Autodesk Inventor part; units mm, degrees
ref_plane "YZ Plane" through (0, 0, 0) normal (1, 0, 0) x (0, 1, 0)
ref_plane "XZ Plane" through (0, 0, 0) normal (0, 1, 0) x (-1, 0, 0)
ref_plane "XY Plane" through (0, 0, 0) normal (0, 0, 1) x (1, 0, 0)
sketch "Sketch1" plane through (0, 0, 0) normal (0, 0, 1) x (1, 0, 0)
  line L0 (0, 0) -> (-42.291, 0)
  line L1 (-42.291, 0) -> (-42.291, 42.291)
  line L2 (-42.291, 42.291) -> (0, 42.291)
  line L3 (0, 42.291) -> (0, 0)
  dimension "d0" = 42.291
  dimension "d1" = 42.291
extrude "Extrusion1" add sketch "Sketch1" along normal blind 42.291
sketch "Sketch2" plane through (0, 0, 42.291) normal (0, 0, 1) x (1, 0, 0)
  line L0 (0, 42.291) -> (-42.291, 42.291)
  line L1 (-42.291, 42.291) -> (-42.291, 0)
  line L2 (-42.291, 0) -> (0, 0)
  line L3 (0, 0) -> (0, 42.291)
  line L4 (-5.6515, 5.6515) -> (-36.6395, 5.6515)
  line L5 (-36.6395, 5.6515) -> (-36.6395, 36.6395)
  line L6 (-36.6395, 36.6395) -> (-5.6515, 36.6395)
  line L7 (-5.6515, 36.6395) -> (-5.6515, 5.6515)
  line L8 (-5.6515, 5.6515) -> (-36.6395, 36.6395) construction
  line L9 (-36.6395, 5.6515) -> (-5.6515, 36.6395) construction
  circle A0 centre (-5.6515, 5.6515) radius 2.794
  circle A1 centre (-36.6395, 5.6515) radius 2.794
  circle A2 centre (-36.6395, 36.6395) radius 2.794
  circle A3 centre (-5.6515, 36.6395) radius 2.794
  point P0 (-21.1455, 21.1455)
  dimension "d4" = 30.988
  dimension "d5" = 30.988
  dimension "d8" = 5.588
  dimension "d9" = 5.588
  dimension "d10" = 5.588
  dimension "d11" = 5.588
extrude "Extrusion2" cut sketch "Sketch2" against normal blind 68.834 contours A1 L5 L4 | L4 L5 A1 | A0 L7 L4 | L4 L7 A0 | A2 L6 L5 | L5 L6 A2 | A3 L6 L7 | L7 L6 A3
sketch "Sketch3" plane through (0, 0, 42.291) normal (0, 0, 1) x (1, 0, 0)
  circle A0 centre (-5.6515, 5.6515) radius 2.794
  circle A1 centre (-5.6515, 36.6395) radius 2.794
  circle A2 centre (-36.6395, 5.6515) radius 2.794
  circle A3 centre (-36.6395, 36.6395) radius 2.794
  line L0 (0, 42.291) -> (-42.291, 42.291)
  line L1 (-42.291, 42.291) -> (-42.291, 0)
  line L2 (-42.291, 0) -> (0, 0)
  line L3 (0, 0) -> (0, 42.291)
  circle A4 centre (-21.1455, 21.1455) radius 2.5019
  dimension "d14" = 5.0038
extrude "Extrusion3" add sketch "Sketch3" along normal blind 24.003 contours A4
properties part number "Nema 17"
For this review, take the finished solid that the model builds, in its own axes (mm). A direction names the side the tool comes from. Give positions to 0.01 mm unless a question says otherwise; leave off trailing zeros. Write each loop counter-clockwise with the first axis right and the second up, starting at its lowest first coordinate (ties: lowest second). Pieces come first, ordered by that corner, then holes. Notation, with made-up numbers: (12.5, 66) -> (63.5, 66) arc R12 cw to (63.5, 74) -> close; hole circle Ø4 at (32, 54.25). An arc over 180 degrees is marked (long way). Use CSV: the item, a comma, the result in double quotes.
Q1. For P1, Ø1, axis at x = -18, z = 59.5, coming from the -Y side; P2, Ø10, axis at x = -36.5, y = 10.5, coming from the +Z side, all flat-tipped, find the tip position at first contact; note any pin that passes through.
Conclusion:
P1,"through"
P2,"z = 42.29"
Q2. Take a section at A-A, the plane x = -38. Write out the cut boundary in (y, z).
Conclusion:
outline,"(0, 0) -> (3.21, 0) -> (3.21, 42.29) -> (0, 42.29) -> close; (8.09, 0) -> (34.2, 0) -> (34.2, 42.29) -> (8.09, 42.29) -> close; (39.08, 0) -> (42.29, 0) -> (42.29, 42.29) -> (39.08, 42.29) -> close"
Q3. Take a section at D-D, the plane x = -15. Write out the cut boundary in (y, z).
Conclusion:
outline,"(0, 0) -> (42.29, 0) -> (42.29, 42.29) -> (0, 42.29) -> close"
Q4. To check wall thickness, follow probe 1 along X at (y, z) = (4, 19); probe 2 along X at (y, z) = (8, 32.5); probe 3 along Y at (x, z) = (-35, 12.5). State the ranges of each line that lie inside material, in increasing order. Write a range as [from, to].
Conclusion:
probe 1,"[-42.29, -38.89], [-34.39, -7.91], [-3.4, 0]"
probe 2,"[-42.29, -38.15], [-35.13, -7.17], [-4.14, 0]"
probe 3,"[0, 3.39], [7.91, 34.38], [38.9, 42.29]"
Q5. Take a section at B-B, the plane y = 7. Write out the cut boundary in (x, z).
Conclusion:
outline,"(-42.29, 0) -> (-39.09, 0) -> (-39.09, 42.29) -> (-42.29, 42.29) -> close; (-34.19, 0) -> (-8.1, 0) -> (-8.1, 42.29) -> (-34.19, 42.29) -> close; (-3.2, 0) -> (0, 0) -> (0, 42.29) -> (-3.2, 42.29) -> close"
Q6. Tool access review of faces 5 (the face through (-23.645, 21.035, 54.124)), 6 (the face through (0, 21, 21)): name each direction out of +Z, -Z, +X, -X, +Y, -Y from which nothing blocks a thin tool from reaching the whole face with its end or side.
Conclusion:
face 5,"+Z"
face 6,"+Z, -Z, +X, +Y, -Y"
Q7. Mouldability with a two-part tool opening along Y and no side actions: class faces 1 (the face through (-6.02, 39.41, 21.44)), 2 (the face through (-21, 0, 21)), 3 (the face through (-38.857, 3.951, 21.442)), 4 (the face through (-26, 21, 42.291)) as pulls with the +Y half, pulls with the -Y half, needs draft (parallel to the pull), parting line crosses it, or undercut.
Conclusion:
face 1,"undercut"
face 2,"pulls with the -Y half"
face 3,"undercut"
face 4,"needs draft"
Q8. Take a section at C-C, the plane z = 34. Write out the cut boundary in (x, y), then the cut area to 3 significant figures.
Conclusion:
outline,"(-42.29, 0) -> (0, 0) -> (0, 42.29) -> (-42.29, 42.29) -> close; hole circle Ø5.59 at (-36.64, 5.65); hole circle Ø5.59 at (-36.64, 36.64); hole circle Ø5.59 at (-5.65, 5.65); hole circle Ø5.59 at (-5.65, 36.64)"
area,"1,690 mm2"
